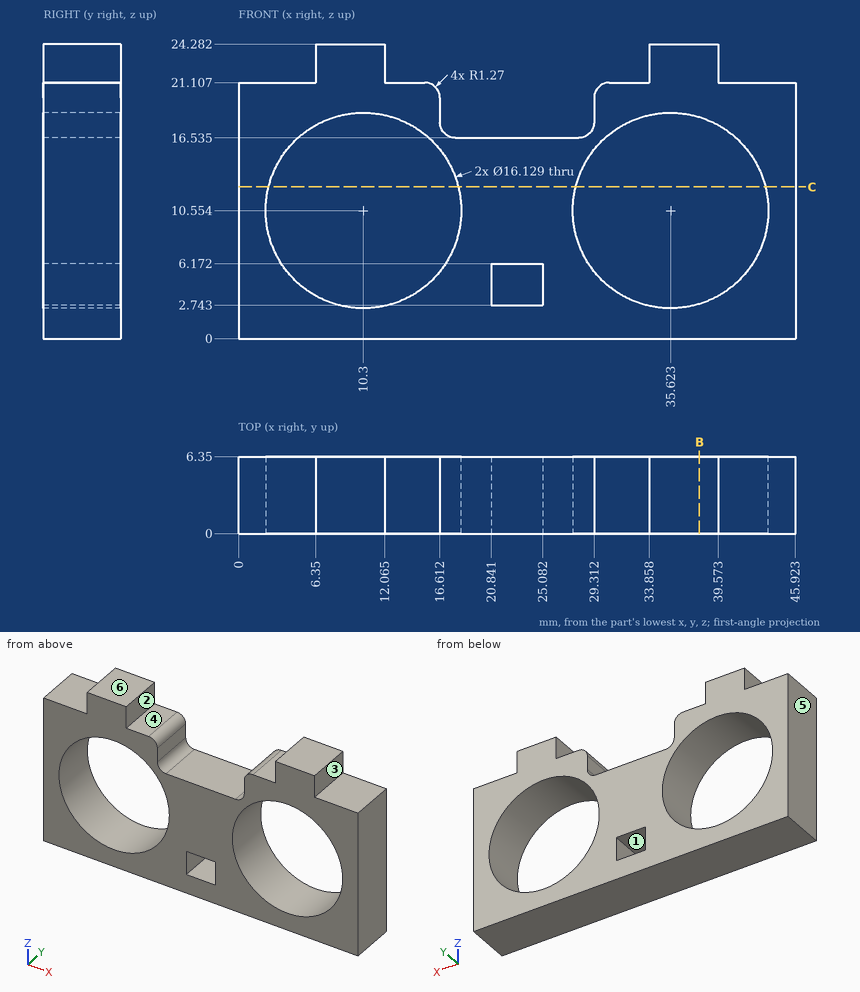
Here's the drawing with two shaded views (mm, measured from the low corner). I have some questions. A direction names the side the tool comes from. Coordinates: 2 decimals unless noted, no trailing zeros. Write each loop counter-clockwise with the first axis right and the second up, starting at its lowest first coordinate (ties: lowest second). Pieces come first, ordered by that corner, then holes. Notation, with made-up numbers: (-21.75, 47.25) - (-8.75, 47.25) arc R10 cw to (-8.75, 64.25) - close; hole circle Ø4 at (37, 23.5). An arc over 180 degrees is marked (long way). Return JSON: item names as keys, results as strings.
Q1. I'm going to push flat-ended pins straight in: pin 1 Ø1.9 at (x, y) = (43, 4) entering from +Z; pin 2 Ø1 at (y, z) = (1.5, 22.5) entering from -X; pin 3 Ø3.5 at (x, y) = (23.5, 3) entering from +Z (1 decimal); pin 4 Ø9.5 at (x, z) = (10.3, 10.55) entering from -Y. Where does each tip first touch, or does it pass through?
Computed values:
{"pin 1": "stops at z = 21.11", "pin 2": "stops at x = 6.35", "pin 3": "stops at z = 16.5", "pin 4": "passes through"}
Q2. If we section it at C-C (z = 12.5): Count the separate pieces of the cut face and the enclosed holes in it.
Computed values:
{"separate pieces": "3", "enclosed holes": "0"}
Q3. On a 3-axis mill with a long thin cutter (end or side, diameter ignored), from which of +Z, -Z, +X, -X, +Y, -Y can I reach the whole of each face in a straight line? I mean the marked faces 1, 2 and 3. Say none if no direction works.
Computed values:
{"face 1": "+Y, -Y", "face 2": "+Z, +Y, -Y", "face 3": "+Z, +X, +Y, -Y"}
Q4. Thinking about a two-plate mould opening in X: for the marked faces 4, 5 and 6, which applies, +X half, -X half, draft (parallel to the pull), parting line (faces both ways), or undercut?
Computed values:
{"face 4": "undercut", "face 5": "-X half", "face 6": "draft"}
Q5. Please list where these lines run through material, in increasing order: L1, parallel to X at y = 1.5, z = 10.75 (1 decimal); L2, parallel to X at y = 5.25, z = 10 (1 decimal); L3, parallel to Z at x = 25, y = 0.75 (1 decimal). Write a range as from..to.
Computed values:
{"L1": "x = 0..2.2, 18.4..27.6, 43.7..45.9", "L2": "x = 0..2.3, 18.3..27.6, 43.7..45.9", "L3": "z = 0..2.7, 6.2..16.5"}
Q6. If we section it at B-B (x = 38): Please give me the cut outline in (y, z).
Computed values:
{"outline": "(0, 0) - (6.35, 0) - (6.35, 2.85) - (0, 2.85) - close; (0, 18.26) - (6.35, 18.26) - (6.35, 24.28) - (0, 24.28) - close"}
